Here's how the part is built. I have some questions about the finished solid (model axes, mm). Face numbers are marked on the shaded views. Round coordinates to 2 decimals unless told otherwise and drop trailing zeros. Write each loop counter-clockwise with the first axis right and the second up, starting at its lowest first coordinate (ties: lowest second). Pieces come first, ordered by that corner, then holes. Notation, with made-up numbers: M 56,52.5 L 65,52.5 A30 cw 65,82.5 Z; hole C -3.5,-37.75 d5. An arc over 180 degrees is marked long. Write item = value, one per line. Start each with the question number.
(1) If we mould it in two halves opening along X, with no side actions, what happens to the marked faces 1, 2 and 3? For each: released by +X, released by -X, zero draft, split by the parting line, or undercut.
(2) I need wall thicknesses on line 1 along X through (y, z) = (5, -6); line 2 along Y through (x, z) = (-7, -4.25); line 3 along X through (y, z) = (6.25, -1.5). Which ranges of each line are inside material? Lowest first, please.
(3) I want a section at A-A (x = -1.5). List the corners of the cut face in (y, z) for me, and give its area (3 significant figures).
(4) Will these pins go through, and if not, where does the flat tip stop? pin 1 Ø6 at (y, z) = (4.5, -12) entering from -X; pin 2 Ø1 at (x, y) = (-10, 7.5) entering from -Z; pin 3 Ø2 at (x, y) = (-6.5, 8) entering from -Z.
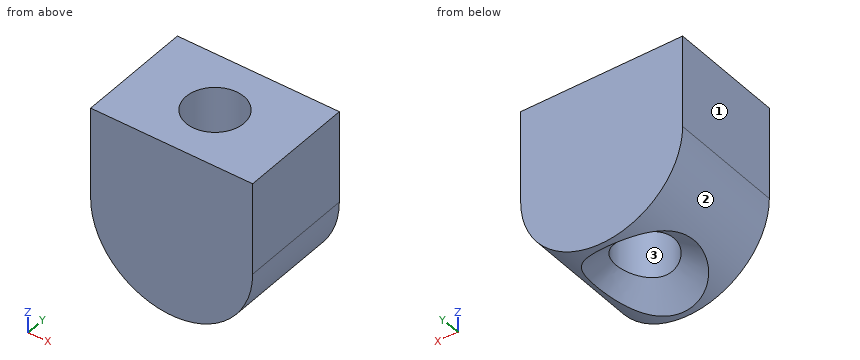
Autodesk Inventor part; units mm, degrees
ref_plane "YZ Plane" through (0, 0, 0) normal (1, 0, 0) x (0, 1, 0)
ref_plane "XZ Plane" through (0, 0, 0) normal (0, 1, 0) x (-1, 0, 0)
ref_plane "XY Plane" through (0, 0, 0) normal (0, 0, 1) x (1, 0, 0)
sketch "Sketch1" plane through (0, 0, 0) normal (0, 1, 0) x (-1, 0, 0)
  line L0 (0, -8) -> (0, 0)
  line L1 (0, 0) -> (14, 0)
  line L2 (14, 0) -> (14, -8)
  arc A0 (0, -8) -> (14, -8) centre (7, -8) ccw
  dimension "d0" = 14
  dimension "d1" = 7
  dimension "d2" = 8
extrude "Extrusion1" add sketch "Sketch1" along normal blind 10
sketch "Sketch2" plane through (-14, 0, 0) normal (0, 0, 1) x (1, 0, 0)
  circle A0 centre (7, 5) radius 2.5
  line L0 (0, 0) -> (14, 0)
  line L1 (0, 0) -> (0, 10)
  dimension "d5" = 5
  dimension "d6" = 5
  dimension "d7" = 7
extrude "Extrusion2" cut sketch "Sketch2" against normal through all
chamfer "Chamfer1" distance 2 angle 45 1 edges at (-9.5, 5.0035, -14.5383)
properties part number "SUPPORT_POULIE"
Returned:
q1.face_1 = released by -X
q1.face_2 = split by the parting line
q1.face_3 = undercut
q2.line_1 = -14 to -9.5, -4.5 to 0
q2.line_2 = 0 to 2.5, 7.5 to 10
q2.line_3 = -14 to -9.17, -4.83 to 0
q3.outline = M 0,-12.33 L 10,-12.33 L 10,0 L 0,0 Z
q3.area = 123 mm²
q4.pin_1 = -13.93
q4.pin_2 = -14.15
q4.pin_3 = -14.51
